Part model, mm, in its own coordinate system. Face numbers are marked on the shaded views. A direction names the side the tool comes from. Round coordinates to 2 decimals unless told otherwise and drop trailing zeros. Write each loop counter-clockwise with the first axis right and the second up, starting at its lowest first coordinate (ties: lowest second). Pieces come first, ordered by that corner, then holes.
```python
from build123d import *

# Parameters (mm, degrees)
ESBO_O2_R                                           = 12.5
RESSALTO_EXTRUS_O1_DEPTH                            = 5
ESBO_O3_R                                           = 4
RESSALTO_EXTRUS_O2_DEPTH                            = 7
ESCAREADO_PARA_PARAFUSO_ALLEN_SEXTAVADO_D           = 3.4
ESCAREADO_PARA_PARAFUSO_ALLEN_SEXTAVADO_CSINK_D     = 6.72
ESCAREADO_PARA_PARAFUSO_ALLEN_SEXTAVADO_CSINK_ANGLE = 90


with BuildPart() as part:
    # Esboço2 → Ressalto-extrusão1 (new body)
    with BuildSketch(Plane.XY):
        Circle(ESBO_O2_R)
    extrude(amount=RESSALTO_EXTRUS_O1_DEPTH)

    # Esboço3 → Ressalto-extrusão2 (add)
    with BuildSketch(Plane.XY.offset(5)):
        Circle(ESBO_O3_R)
    extrude(amount=RESSALTO_EXTRUS_O2_DEPTH)

    # Escareado para parafuso Allen sextavado escareado de M31 (through all)
    with Locations(Plane.XY.offset(5)):
        with Locations((0, 8), (8, 0), (0, -8), (-8, 0)):
            CounterSinkHole(ESCAREADO_PARA_PARAFUSO_ALLEN_SEXTAVADO_D / 2, ESCAREADO_PARA_PARAFUSO_ALLEN_SEXTAVADO_CSINK_D / 2, counter_sink_angle=ESCAREADO_PARA_PARAFUSO_ALLEN_SEXTAVADO_CSINK_ANGLE)


solid = part.part
```
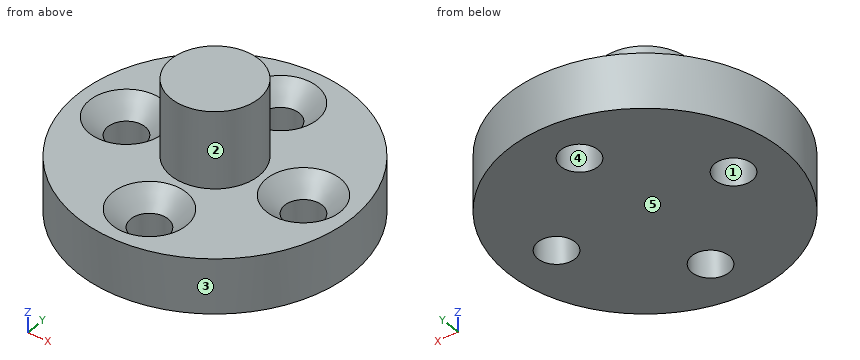
Q1. Mould opens along X. For the marked faces 3, 4 and 5 say: +X half, -X half, draft (parallel to the pull), parting line (faces both ways), or undercut.
Values follow:
face 3: parting line
face 4: undercut
face 5: draft
Q2. Cut at C-C on z = 4.5. Write the cut outline in (x, y), plus the area to 3 significant figures.
Values follow:
outline: circle Ø25 at (0, 0); hole circle Ø5.72 at (-8, 0); hole circle Ø5.72 at (0, -8); hole circle Ø5.72 at (0, 8); hole circle Ø5.72 at (8, 0)
area: 388 mm2
Q3. Cut at A-A on x = 0. Write the cut outline in (y, z), plus the area to 3 significant figures.
Values follow:
outline: (-12.5, 0) - (-9.7, 0) - (-9.7, 3.34) - (-11.36, 5) - (-12.5, 5) - close; (-6.3, 0) - (6.3, 0) - (6.3, 3.34) - (4.64, 5) - (4, 5) - (4, 12) - (-4, 12) - (-4, 5) - (-4.64, 5) - (-6.3, 3.34) - close; (9.7, 0) - (12.5, 0) - (12.5, 5) - (11.36, 5) - (9.7, 3.34) - close
area: 141 mm2
Q4. Cut at D-D on x = -8. Write the cut outline in (y, z).
Values follow:
outline: (-9.6, 0) - (-1.7, 0) - (-1.7, 3.34) - (-3.36, 5) - (-9.6, 5) - close; (1.7, 0) - (9.6, 0) - (9.6, 5) - (3.36, 5) - (1.7, 3.34) - close
Q5. Wall check: L1, parallel to Y at x = 0, z = 1.25; L2, parallel to Y at x = -1.5, z = 3; L3, parallel to Z at x = -8, y = 8.25. Give the ranges that are in metal, low to high.
Values follow:
L1: y = -12.5 to -9.7, -6.3 to 6.3, 9.7 to 12.5
L2: y = -12.41 to -8.8, -7.2 to 7.2, 8.8 to 12.41
L3: z = 0 to 5
Q6. Drop flat-ended pins along their axis: pin 1 (3 mm diameter, centred on x = 0, y = -8, fed in from -Z); pin 2 (3 mm diameter, centred on x = -1.5, z = 10.5, fed in from -Y); pin 3 (5.5 mm diameter, centred on x = 8, y = 0, fed in from +Z); pin 4 (4 mm diameter, centred on x = -8, y = 0, fed in from +Z). Give the stop position or say it passes through.
Values follow:
pin 1: passes through
pin 2: stops at y = -4
pin 3: stops at z = 4.39
pin 4: stops at z = 3.64
Q7. Which spindle directions (+Z, -Z, +X, -X, +Y, -Y) get a long thin tool onto all of the face, cutting with end or side? Do the marked faces 1 and 2. Say none if no direction does.
Values follow:
face 1: +Z, -Z
face 2: +Z
